from build123d import *

# Parameters (mm, degrees)
SKETCH2_R           = 9.525
BOSS_EXTRUDE1_DEPTH = 6.35
SKETCH2_3_R         = 25.4
SKETCH2_3_R_2       = 12.7
BOSS_EXTRUDE2_DEPTH = 19.05
SKETCH3_R           = 9.525
BOSS_EXTRUDE3_DEPTH = 12.7


with BuildPart() as part:
    # Sketch2 → Boss-Extrude1 (new body, symmetric)
    with BuildSketch(Plane.XY):
        with BuildLine():
            ThreePointArc((25.4, 0), (8.980256121, -23.759524406), (-19.05, -16.800520825))
            Line((-19.05, -16.800520825), (-19.05, -50.8))
            ThreePointArc((-19.05, -50.8), (-13.470384182, -64.270384182), (0, -69.85))
            Line((0, -69.85), (69.85, -69.85))
            ThreePointArc((69.85, -69.85), (95.25, -44.45), (69.85, -19.05))
            Line((69.85, -19.05), (44.45, -19.05))
            ThreePointArc((44.45, -19.05), (30.979615818, -13.470384182), (25.4, 0))
        make_face()
        with Locations((0, -44.45)):
            Circle(SKETCH2_R, mode=Mode.SUBTRACT)
        with Locations((69.85, -44.45)):
            Circle(SKETCH2_R, mode=Mode.SUBTRACT)
    extrude(amount=BOSS_EXTRUDE1_DEPTH, both=True)

    # Sketch2_3 → Boss-Extrude2 (add, symmetric)
    with BuildSketch(Plane.XY):
        Circle(SKETCH2_3_R)
        Circle(SKETCH2_3_R_2, mode=Mode.SUBTRACT)
    extrude(amount=BOSS_EXTRUDE2_DEPTH, both=True)

    # Sketch3 → Boss-Extrude3 (add)
    with BuildSketch(Plane.XZ.offset(69.85)):
        with BuildLine():
            Line((19.05, -31.75), (19.05, 31.75))
            ThreePointArc((19.05, 31.75), (38.1, 50.8), (57.15, 31.75))
            Line((57.15, 31.75), (57.15, -31.75))
            ThreePointArc((57.15, -31.75), (38.1, -50.8), (19.05, -31.75))
        make_face()
        with Locations((38.1, 31.75)):
            Circle(SKETCH3_R, mode=Mode.SUBTRACT)
        with Locations((38.1, -31.75)):
            Circle(SKETCH3_R, mode=Mode.SUBTRACT)
    extrude(amount=-BOSS_EXTRUDE3_DEPTH)


solid = part.part
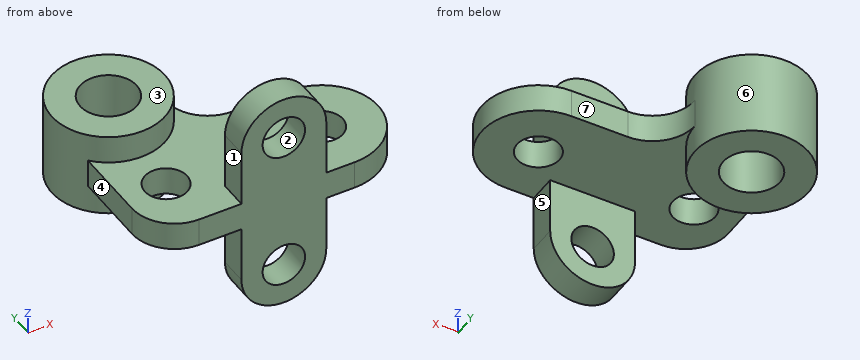
Input: part model. Units: mm. Frame: model coordinates. Face numbers are marked on the shaded views. A direction names the side the tool comes from. Give positions to 0.01 mm unless a question says otherwise; leave off trailing zeros. Loops run counter-clockwise (first coordinate to the right, second up) from the corner with the lowest first, then second, coordinate; pieces in that order, holes last. Notation, with made-up numbers: (-15, -10.5) -> (39, -10.5) arc R13 cw to (39, 7.5) -> close; hole circle Ø3 at (-8, 22.5). An arc over 180 degrees is marked (long way). Answer as a JSON object with one key per item and string values. Group by question number.
Item 1: Pull-direction query (Z, two-part tool) for the marked faces 1, 2 and 3; classes: released by +Z, released by -Z, zero draft, split by the parting line, or undercut.
Item 2: Cut plane A-A, the plane z = 11.5. Return the cut outline in (x, y).
Item 3: Cut plane D-D, the plane z = 30. Return the cut outline in (x, y).
Item 4: Pin query (flat end, axial travel): P1, Ø10, axis at y = -61, z = 14, coming from the +X side; P2, Ø10, axis at x = 68.5, y = -20.5, coming from the -Z side; P3, Ø21, axis at x = 47, y = -38.5, coming from the +Z side; P4, Ø17, axis at x = 0, y = -44.45, coming from the -Z side. Return the tip coordinate at first contact, or that it passes through.
Item 5: Cut plane C-C, the plane x = -3. Return the cut outline in (y, z), and give its area (3 significant figures).
Item 6: Cut plane B-B, the plane y = -44.45. Return the cut outline in (x, z) (3 decimals), and give its area (3 significant figures).
Item 7: Reachability of the marked faces 4, 5, 6 and 7 from +Z, -Z, +X, -X, +Y, -Y: full face, straight path, thin tool, end or side. Return the list, or none.
Item 8: Line query: probe 1 along Y at (x, z) = (0, -3) (3 decimals); probe 2 along X at (y, z) = (-44, 1); probe 3 along Z at (x, y) = (38.1, -65.25) (3 decimals). Output: solid intervals per line, ascending.
Checks:
{
 "1": {"face 1": "zero draft", "face 2": "undercut", "face 3": "released by +Z"},
 "2": {"outline": "circle Ø50.8 at (0, 0); (19.05, -69.85) -> (57.15, -69.85) -> (57.15, -57.15) -> (19.05, -57.15) -> close; hole circle Ø25.4 at (0, 0)"},
 "3": {"outline": "(19.05, -69.85) -> (28.74, -69.85) -> (28.74, -57.15) -> (19.05, -57.15) -> close; (47.46, -69.85) -> (57.15, -69.85) -> (57.15, -57.15) -> (47.46, -57.15) -> close"},
 "4": {"P1": "stops at x = 57.15", "P2": "stops at z = -6.35", "P3": "stops at z = 6.35", "P4": "passes through"},
 "5": {"outline": "(-69.61, -6.35) -> (-53.49, -6.35) -> (-53.49, 6.35) -> (-69.61, 6.35) -> close; (-35.41, -6.35) -> (-25.22, -6.35) -> (-25.22, -19.05) -> (-12.34, -19.05) -> (-12.34, 19.05) -> (-25.22, 19.05) -> (-25.22, 6.35) -> (-35.41, 6.35) -> close; (12.34, -19.05) -> (25.22, -19.05) -> (25.22, 19.05) -> (12.34, 19.05) -> close", "area": "1,320 mm²"},
 "6": {"outline": "(-19.05, -6.35) -> (-9.525, -6.35) -> (-9.525, 6.35) -> (-19.05, 6.35) -> close; (9.525, -6.35) -> (60.325, -6.35) -> (60.325, 6.35) -> (9.525, 6.35) -> close; (79.375, -6.35) -> (95.25, -6.35) -> (95.25, 6.35) -> (79.375, 6.35) -> close", "area": "968 mm²"},
 "7": {"face 4": "+Z, -Z, -X, -Y", "face 5": "-Z, +X, +Y, -Y", "face 6": "none", "face 7": "+Z, -Z, +X, +Y"},
 "8": {"probe 1": "y = -69.85 to -53.975, -34.925 to -12.7, 12.7 to 25.4", "probe 2": "x = -19.05 to -9.51, 9.51 to 60.34, 79.36 to 95.25", "probe 3": "z = -50.8 to -41.275, -22.225 to 22.225, 41.275 to 50.8"}
}
